```python
from build123d import *

# Parameters (mm, degrees)
F0_W     = 50.8
F0_H     = 76.2
F0_W_2   = 47.625
F0_H_2   = 73.025
F1_DEPTH = 1016
F2_W     = 53.975
F2_H     = 152.4
F3_DEPTH = 1.5875
F4_R     = 7.9375
F5_DEPTH = 1.5875


with BuildPart() as f1:
    # F0 (on Front) → F1 (new body)
    with BuildSketch(Plane.XZ):
        with Locations((25.4, 38.1)):
            Rectangle(F0_W, F0_H)
        with Locations((25.4, 38.1)):
            Rectangle(F0_W_2, F0_H_2, mode=Mode.SUBTRACT)
    extrude(amount=-F1_DEPTH)

    # F2 (on face) → F3 (join)
    with BuildSketch(Plane.XZ):
        with Locations((25.4, 38.1)):
            Rectangle(F2_W, F2_H)
    extrude(amount=F3_DEPTH)

    # F4 (on face) → F5 (cut, through all)
    with BuildSketch(Plane.XZ.offset(1.5875)):
        with Locations((25.4, 95.25)):
            Circle(F4_R)
        with Locations((25.4, -19.05)):
            Circle(F4_R)
    extrude(amount=-F5_DEPTH, mode=Mode.SUBTRACT)


solid = f1.part
```
CAD build for the part. Positions are in the model's coordinates, mm. A direction names the side the tool comes from. Round coordinates to 2 decimals unless told otherwise and drop trailing zeros. Order: outer loops, then holes, each group sorted by start corner. A loop starts at its lowest first (then second) coordinate and runs counter-clockwise, first axis right, second up.
Q1. Wall check: L1, parallel to Z at x = 25.4, y = -1.15; L2, parallel to Z at x = 48, y = 143; L3, parallel to X at y = 588, z = 62.5. Give the ranges that are in metal, low to high.
Q2. Drop flat-ended pins along their axis: pin 1 (1.5 mm diameter, centred on x = 22, z = 68, fed in from +Y); pin 2 (3 mm diameter, centred on x = 37.5, y = 658, fed in from +Z); pin 3 (3 mm diameter, centred on y = 356, z = 44.5, fed in from +X). Give the stop position or say it passes through.
Q3. Slice it at A-A (y = 510.5). Write the cut outline in (x, z).
Q4. Slice it at B-B (z = 36). Write the cut outline in (x, y).
Q5. Two-plate mould, pull along X, no slides. Class faces 4 (the cylindrical face through (24.37, -0.8, 103.12)), 5 (the flat face through (0, 501, 38)), 6 (the flat face through (50.8, 501, 38)), 7 (the flat face through (25, 501, 76.2)): pulls with the +X half, pulls with the -X half, needs draft (parallel to the pull), parting line crosses it, or undercut.
Q6. Which spindle directions (+Z, -Z, +X, -X, +Y, -Y) get a long thin tool onto all of the face, cutting with end or side? Do faces 1 (the flat face through (25, 501, 0)), 2 (the flat face through (25, 501, 74.613)), 3 (the flat face through (25, -1.588, 39)). Say none if no direction does.
Results below:
1. L1: z = -38.1 to -26.99, -11.11 to 87.31, 103.19 to 114.3
1. L2: z = 0 to 1.59, 74.61 to 76.2
1. L3: x = 0 to 1.59, 49.21 to 50.8
2. pin 1: stops at y = 0
2. pin 2: stops at z = 76.2
2. pin 3: stops at x = 50.8
3. outline: (0, 0) - (50.8, 0) - (50.8, 76.2) - (0, 76.2) - close; hole (1.59, 1.59) - (49.21, 1.59) - (49.21, 74.61) - (1.59, 74.61) - close
4. outline: (-1.59, -1.59) - (52.39, -1.59) - (52.39, 0) - (50.8, 0) - (50.8, 1016) - (49.21, 1016) - (49.21, 0) - (1.59, 0) - (1.59, 1016) - (0, 1016) - (0, 0) - (-1.59, 0) - close
5. face 4: undercut
5. face 5: pulls with the -X half
5. face 6: pulls with the +X half
5. face 7: needs draft
6. face 1: -Z, +X, -X, +Y
6. face 2: +Y
6. face 3: +Z, -Z, +X, -X, -Y
